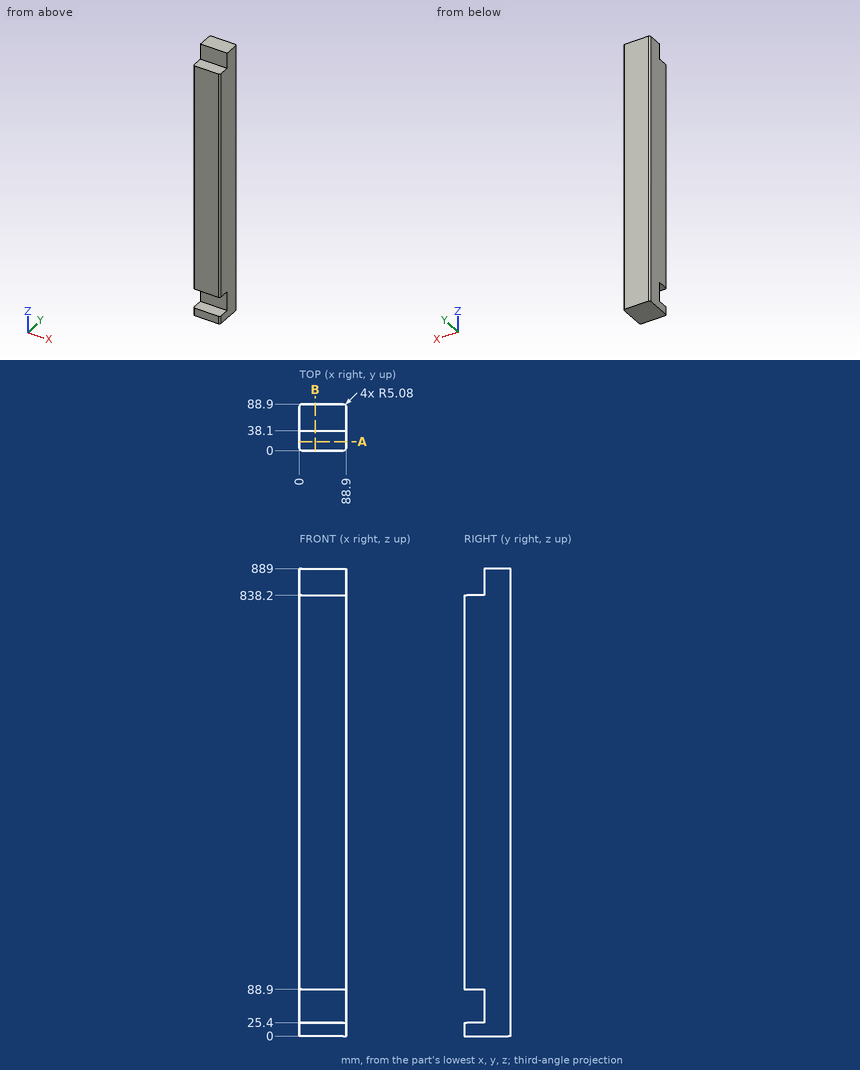
Study the drawing (mm; zero at the part's minimum x, y, z) and answer. Give positions to 0.01 mm unless a question says otherwise; leave off trailing zeros. Loops run counter-clockwise (first coordinate to the right, second up) from the corner with the lowest first, then second, coordinate; pieces in that order, holes last. Notation, with made-up numbers: M 85,48.5 L 130,48.5 A13 cw 130,58.5 Z; hole C 4,-2 d7. An arc over 180 degrees is marked long. Answer as CSV lines item,"result".
Item 1: The part is cut by section B-B (x = 30). Give the vertices of the cut face in (y, z), and give its area (3 significant figures).
Values follow:
outline,"M 0,0 L 88.9,0 L 88.9,889 L 38.1,889 L 38.1,838.2 L 0,838.2 L 0,88.9 L 38.1,88.9 L 38.1,25.4 L 0,25.4 Z"
area,"74,700 mm^2"
Item 2: Straight lines are drawn through the part: line 1 along Z through (x, y) = (57.5, 30); line 2 along X through (y, z) = (5, 678.5). For each, find the intervals that lie inside material, in ascending order. Write a range as [from, to].
Values follow:
line 1,"z = [0, 25.4], [88.9, 838.2]"
line 2,"x = [0, 88.9]"
Item 3: The part is cut by section A-A (y = 17.5). Give the vertices of the cut face in (x, z).
Values follow:
outline,"M 0,0 L 88.9,0 L 88.9,25.4 L 0,25.4 Z; M 0,88.9 L 88.9,88.9 L 88.9,838.2 L 0,838.2 Z"
Item 4: Given pin 1 Ø4 at (x, y) = (79, 35.5) entering from +Z; pin 2 Ø19 at (x, z) = (53, 49.5) entering from -Y, each flat-ended and moving along its own axis, determine where each tip first touches the part or whether it passes through.
Values follow:
pin 1,"stops at z = 838.2"
pin 2,"stops at y = 38.1"
